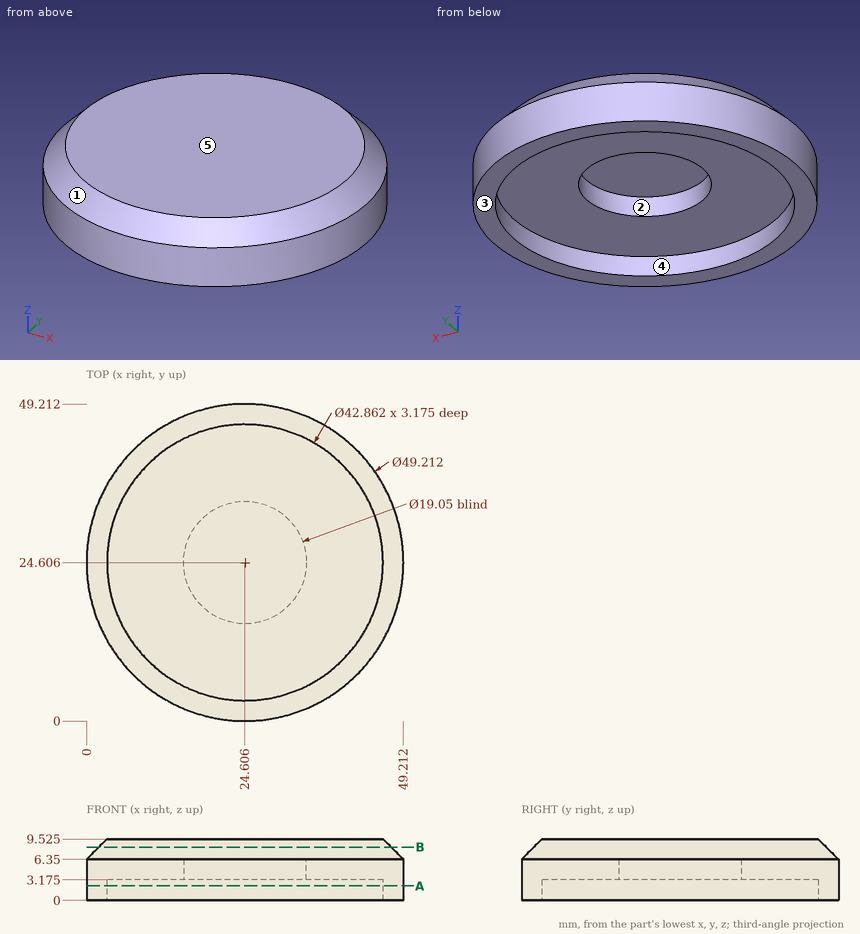
Part print with two shaded views. Sizes in mm from the minimum x, y, z corner. A direction names the side the tool comes from. Coordinates: 2 decimals unless noted, no trailing zeros. Write each loop counter-clockwise with the first axis right and the second up, starting at its lowest first coordinate (ties: lowest second). Pieces come first, ordered by that corner, then holes. Notation, with made-up numbers: (-19, 80.5) -> (36, 80.5) arc R24 ccw to (36, 92.5) -> close; hole circle Ø9 at (75, -9). An arc over 180 degrees is marked (long way). Return JSON: item names as keys, results as strings. Group by question number.
Q1. Drill centre lines: line 1 (X direction, y = 25, z = 5.75); line 2 (Z direction, x = 45.5, y = 21) (1 decimal); line 3 (Y direction, x = 43.5, z = 2.5) (1 decimal). Where is each one in solid material? Low to high.
Q2. Flat gauge pins, fed straight in: pin 1 (21 mm diameter, centred on x = 20.5, y = 23.5, fed in from -Z) (1 decimal); pin 2 (11.5 mm diameter, centred on x = 24.61, y = 24.61, fed in from -Z); pin 3 (1 mm diameter, centred on x = 20, z = 3, fed in from +Y). Where does each tip first touch, or does it go through?
Q3. Pull direction Y, two halves, no side cores. Call the marked faces 1, 2 and 3: released by +Y, released by -Y, zero draft, split by the parting line, or undercut.
Q4. Cut at B-B, the plane z = 8.25. Give the cut face in (x, y), then the cut area to 3 significant figures.
Q5. Cut at A-A, the plane z = 2.25. Give the cut face in (x, y).
Q6. Which spindle directions (+Z, -Z, +X, -X, +Y, -Y) get a long thin tool onto all of the face, cutting with end or side? Do the marked faces 4 and 5. Say none if no direction does.
Returned:
{
 "1": {"line 1": "x = 0 to 15.09, 34.12 to 49.21", "line 2": "z = 3.2 to 9.5", "line 3": "y = 8.8 to 14.5, 34.7 to 40.4"},
 "2": {"pin 1": "stops at z = 3.2", "pin 2": "stops at z = 6.35", "pin 3": "stops at y = 48.87"},
 "3": {"face 1": "split by the parting line", "face 2": "undercut", "face 3": "zero draft"},
 "4": {"outline": "circle Ø45.41 at (24.61, 24.61)", "area": "1,620 mm2"},
 "5": {"outline": "circle Ø49.21 at (24.61, 24.61); hole circle Ø42.86 at (24.61, 24.61)"},
 "6": {"face 4": "-Z", "face 5": "+Z, +X, -X, +Y, -Y"}
}
